Could you check a few things on this drawing? It's one solid part, dimensions in mm from its lowest x, y, z. A direction names the side the tool comes from. Round coordinates to 2 decimals unless told otherwise and drop trailing zeros. Write each loop counter-clockwise with the first axis right and the second up, starting at its lowest first coordinate (ties: lowest second). Pieces come first, ordered by that corner, then holes. Notation, with made-up numbers: (-21.5, -32.75) -> (7.5, -32.75) arc R18 ccw to (7.5, -13.75) -> close; hole circle Ø7 at (-14.5, -35.5). An arc over 180 degrees is marked (long way). Answer in a Markdown table with one row per item.
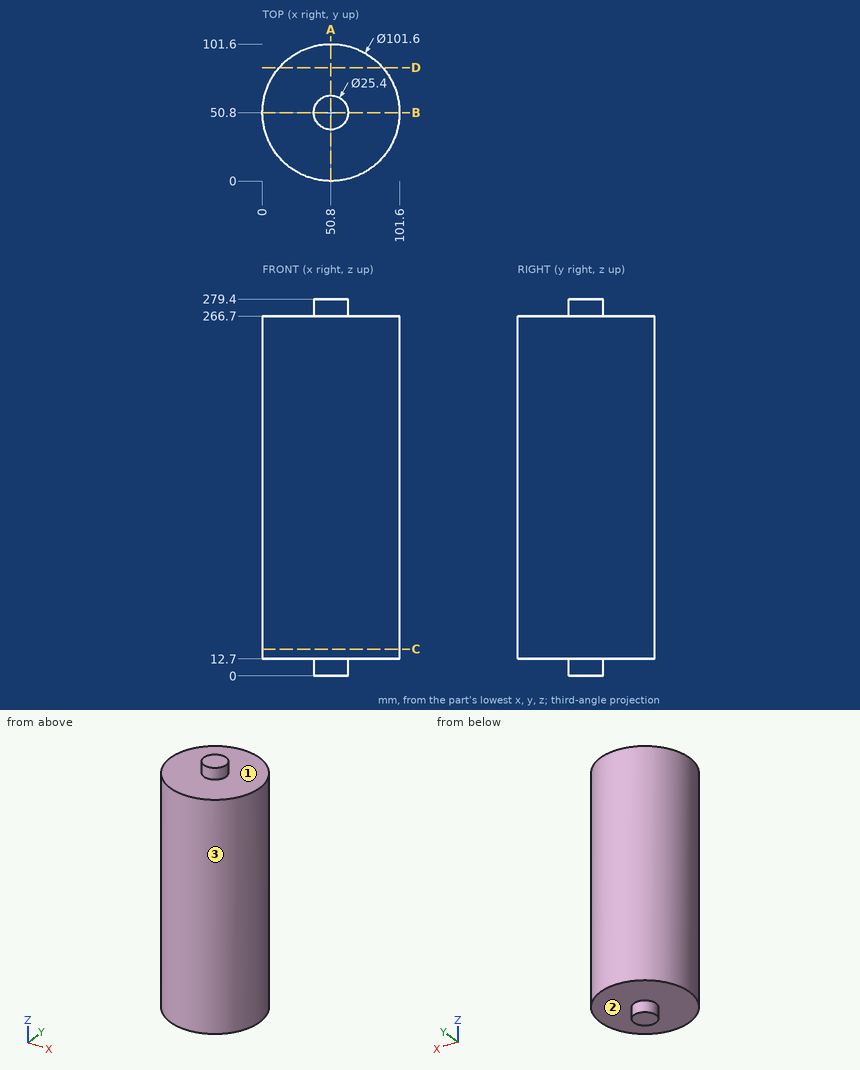
1) I need wall thicknesses on line 1 (X direction, y = 53, z = 251); line 2 (X direction, y = 52, z = 131); line 3 (Z direction, x = 16, y = 76). Which ranges of each line are inside material? Lowest first, please. Write a range as [from, to].
Response:
| item | result |
|---|---|
| line 1 | x = [0.05, 101.55] |
| line 2 | x = [0.01, 101.59] |
| line 3 | z = [12.7, 266.7] |
2) I want a section at A-A, the plane x = 50.8. List the corners of the cut face in (y, z) for me.
Response:
| item | result |
|---|---|
| outline | (0, 12.7) -> (38.1, 12.7) -> (38.1, 0) -> (63.5, 0) -> (63.5, 12.7) -> (101.6, 12.7) -> (101.6, 266.7) -> (63.5, 266.7) -> (63.5, 279.4) -> (38.1, 279.4) -> (38.1, 266.7) -> (0, 266.7) -> close |
3) Which directions (+Z, -Z, +X, -X, +Y, -Y) give clear straight access to the entire face, cutting with the end or side of a thin tool? Please do the marked faces 1, 2 and 3.
Response:
| item | result |
|---|---|
| face 1 | +Z |
| face 2 | -Z |
| face 3 | +Z, -Z |
4) For pin 1 (8 mm diameter, centred on x = 42, z = 68, fed in from +Y); pin 2 (4 mm diameter, centred on x = 15.5, z = 218, fed in from -Y); pin 3 (10 mm diameter, centred on y = 58, z = 115, fed in from +X), each with a flat end and sliding along its axis, tell me the tip position at first contact or that it passes through.
Response:
| item | result |
|---|---|
| pin 1 | stops at y = 101.37 |
| pin 2 | stops at y = 12.44 |
| pin 3 | stops at x = 101.55 |
5) I want a section at D-D, the plane y = 84. List the corners of the cut face in (x, z) for me, and give its area (3 significant figures).
Response:
| item | result |
|---|---|
| outline | (12.35, 12.7) -> (89.25, 12.7) -> (89.25, 266.7) -> (12.35, 266.7) -> close |
| area | 19,500 mm^2 |
6) I want a section at C-C, the plane z = 20. List the corners of the cut face in (x, y) for me, and give its area (3 significant figures).
Response:
| item | result |
|---|---|
| outline | circle Ø101.6 at (50.8, 50.8) |
| area | 8,110 mm^2 |
